```python
from build123d import *

# Parameters (mm, degrees)
F0_R     = 114.3
F2_DEPTH = 1.016
F1_R     = 76.2
F3_DEPTH = 10.16
F5_DEPTH = 25.4


with BuildPart() as f2:
    # F0 (on Top) → F2 (new body)
    with BuildSketch(Plane.XY):
        Circle(F0_R)
    extrude(amount=F2_DEPTH)

    # F1 (on Top) → F3 (join)
    with BuildSketch(Plane.XY):
        Circle(F1_R)
    extrude(amount=F3_DEPTH)

    # F4 (on Top) → F5 (cut)
    with BuildSketch(Plane.XY):
        Polygon((7.3323484187, 0), (3.6661742094, 6.35), (-3.6661742094, 6.35), (-7.3323484187, 0), (-3.6661742094, -6.35), (3.6661742094, -6.35), align=None)
    extrude(amount=F5_DEPTH, mode=Mode.SUBTRACT)


solid = f2.part
```
Check sheet for the modelled part. Datum: model origin and axes. Units: mm. A direction names the side the tool comes from. Give positions to 0.01 mm unless a question says otherwise; leave off trailing zeros. Loops run counter-clockwise (first coordinate to the right, second up) from the corner with the lowest first, then second, coordinate; pieces in that order, holes last. Notation, with made-up numbers: M 36.5,0.5 L 52.5,0.5 A34 ccw 52.5,30.5 Z; hole C 51.5,40 d11. An arc over 180 degrees is marked long. Answer in a Markdown table with one row per item.
1) Depth check by flat-ended pin: pin 1 (6 mm diameter, centred on x = -52.5, y = -89, fed in from +Z); pin 2 (10 mm diameter, centred on x = 66.5, y = 14, fed in from -Z); pin 3 (3 mm diameter, centred on x = 40, z = 7.5, fed in from +Y); pin 4 (6 mm diameter, centred on x = 45.5, z = 7, fed in from -Y). Enter the tip coordinate at first touch or a pass-through.
Solutions:
| item | result |
|---|---|
| pin 1 | stops at z = 1.02 |
| pin 2 | stops at z = 0 |
| pin 3 | stops at y = 65.76 |
| pin 4 | stops at y = -63.25 |
2) Cross-section at A-A (x = 0). Enter the section's corners in (y, z), plus the area to 3 significant figures.
Solutions:
| item | result |
|---|---|
| outline | M -114.3,0 L -6.35,0 L -6.35,10.16 L -76.2,10.16 L -76.2,1.02 L -114.3,1.02 Z; M 6.35,0 L 114.3,0 L 114.3,1.02 L 76.2,1.02 L 76.2,10.16 L 6.35,10.16 Z |
| area | 1,500 mm^2 |
3) Mould release check, pull along X, two halves, no side actions. Record for faces 4 (the face through (-60.47, -46.367, 5.524)), 5 (the face through (16, 1, 10.16)), 6 (the face through (0, 6.35, 5)): released by +X, released by -X, zero draft, split by the parting line, or undercut.
Solutions:
| item | result |
|---|---|
| face 4 | split by the parting line |
| face 5 | zero draft |
| face 6 | undercut |
4) Cross-section at B-B (y = -3). Enter the section's corners in (x, z).
Solutions:
| item | result |
|---|---|
| outline | M -114.26,0 L -5.6,0 L -5.6,10.16 L -76.14,10.16 L -76.14,1.02 L -114.26,1.02 Z; M 5.6,0 L 114.26,0 L 114.26,1.02 L 76.14,1.02 L 76.14,10.16 L 5.6,10.16 Z |
5) Cross-section at D-D (x = 58.5). Enter the section's corners in (y, z), plus the area to 3 significant figures.
Solutions:
| item | result |
|---|---|
| outline | M -98.19,0 L 98.19,0 L 98.19,1.02 L 48.83,1.02 L 48.83,10.16 L -48.83,10.16 L -48.83,1.02 L -98.19,1.02 Z |
| area | 1,090 mm^2 |
6) Cross-section at C-C (z = 4.25). Enter the section's corners in (x, y), plus the area to 3 significant figures.
Solutions:
| item | result |
|---|---|
| outline | C 0,0 d152.4; hole M -7.33,0 L -3.67,-6.35 L 3.67,-6.35 L 7.33,0 L 3.67,6.35 L -3.67,6.35 Z |
| area | 18,100 mm^2 |
7) Thickness scan on line 1 (Z direction, x = -96, y = 7); line 2 (X direction, y = 5.5, z = 6.5); line 3 (Y direction, x = -44, z = 8.75). Record the ranges inside material, lowest first.
Solutions:
| item | result |
|---|---|
| line 1 | z = 0 to 1.02 |
| line 2 | x = -76 to -4.16, 4.16 to 76 |
| line 3 | y = -62.21 to 62.21 |
8) Tool access check on faces 1 (the face through (24, -75, 1.016)), 2 (the face through (-2, -24, 0)), 3 (the face through (-5.474, 3.219, 5.009)). Record the directions out of +Z, -Z, +X, -X, +Y, -Y that give a thin tool (end or side, any length) a straight path to the whole face; none if there is none.
Solutions:
| item | result |
|---|---|
| face 1 | +Z |
| face 2 | -Z, +X, -X, +Y, -Y |
| face 3 | +Z, -Z |
